Can you work these out from the model? Positions are in its coordinate system, mm. A direction names the side the tool comes from. Round coordinates to 2 decimals unless told otherwise and drop trailing zeros. Write each loop counter-clockwise with the first axis right and the second up, starting at its lowest first coordinate (ties: lowest second). Pieces come first, ordered by that corner, then holes. Notation, with made-up numbers: (2.5, 52.25) -> (39.5, 52.25) arc R11 cw to (39.5, 64.25) -> close; hole circle Ø10 at (50, 73). An arc over 180 degrees is marked (long way). Write item = value, one per line. Start each with the question number.
1) Imagine slicing it at B-B, the plane z = 0.9. State how many separate pieces and enclosed holes the cut face has, then the cut area to 3 significant figures.
2) If I drill on line 1 (Y direction, x = -1, z = 0.1); line 2 (Y direction, x = -15, z = 1.35); line 3 (Y direction, x = 9.25, z = 0.4), over which ranges is the centre line in solid material (lowest first)?
3) Imagine slicing it at A-A, the plane y = -13. Please give me the cut outline in (x, z) (3 decimals).
4) For faces 4 (the face through (8.4, -13.7, 1)), 5 (the face through (-0.2, -22.5, 1)), 6 (the face through (11.4, -12.7, 1)), which set-ups out of +Z, -Z, +X, -X, +Y, -Y let a thin tool reach every point of the face, with its end or its side?
5) I'm going to push flat-ended pins straight in: pin 1 (5 mm diameter, centred on x = -4, y = -16, fed in from +Z); pin 2 (3 mm diameter, centred on x = -15, y = -20, fed in from -Z). Where does each tip first touch, or does it pass through?
6) Thinking about a two-plate mould opening in X: for faces 1 (the face through (8.06, -0.91, 0.99)), 2 (the face through (-11.328, -12.604, 0.986)), 3 (the face through (0, -10, 0)), which applies, +X half, -X half, draft (parallel to the pull), parting line (faces both ways), or undercut?
from build123d import *

# Parameters (mm, degrees)
SKETCH_1_R         = 3
SKETCH_1_R_2       = 1
EXTRUDE_1_DEPTH    = 2
EXTRUDE_1_2_DEPTH  = 2
SKETCH_1_RX        = 12
SKETCH_1_RY        = 10.5
SKETCH_1_R_3       = 7.5
SKETCH_1_R_4       = 1.5
EXTRUDE_1_3_DEPTH  = 2
EXTRUDE_START      = -2
EXTRUDE_3_DEPTH    = 2
FILLET_3_R         = 1
EXTRUDE_4_DEPTH    = 2
HOLE_WIZARD_M3_1_D = 2.5


with BuildPart() as part:
    # Sketch 1 → Extrude 1 (new body)
    with BuildSketch(Plane.XY):
        with Locations((-15, -20)):
            Circle(SKETCH_1_R)
        with Locations((-15, -20)):
            Circle(SKETCH_1_R_2, mode=Mode.SUBTRACT)
    extrude(amount=EXTRUDE_1_DEPTH)



with BuildPart() as body_2:
    # Sketch 1 → Extrude 1 2 (new body)
    with BuildSketch(Plane.XY):
        with Locations(Location((15, -20, 0), (0, 0, 180))):
            Circle(SKETCH_1_R)
        with Locations(Location((15, -20, 0), (0, 0, 180))):
            Circle(SKETCH_1_R_2, mode=Mode.SUBTRACT)
    extrude(amount=EXTRUDE_1_2_DEPTH)


with BuildPart() as body_3:
    # Sketch 1 → Extrude 1 3 (new body)
    with BuildSketch(Plane.XY):
        with Locations((0, 0)):
            Ellipse(SKETCH_1_RX, SKETCH_1_RY)
        Circle(SKETCH_1_R_3, mode=Mode.SUBTRACT)
        with Locations((9.25, 0)):
            Circle(SKETCH_1_R_4, mode=Mode.SUBTRACT)
        with Locations(Location((-9.25, 0, 0), (0, 0, 180))):
            Circle(SKETCH_1_R_4, mode=Mode.SUBTRACT)
    extrude(amount=EXTRUDE_1_3_DEPTH)


with BuildPart() as part_1:
    add(part.part)

    add(body_2.part)  # Extrude 3 merges body 2

    add(body_3.part)  # Extrude 3 merges body 3
    # Sketch 7 → Extrude 3 (add)
    with BuildSketch(Plane.XY.offset(2).offset(EXTRUDE_START)):
        with BuildLine():
            Line((-7.838039348, -7.95071913), (-14.641154273, -17.021539031))
            ThreePointArc((-14.641154273, -17.021539031), (-13.2, -17.6), (-12.241154273, -18.821539031))
            Line((-12.241154273, -18.821539031), (-5.216878938, -9.455838584))
            add(Edge.make_bspline(
                [(-7.838039348, -7.95071913), (-6.640783086, -8.854377448), (-5.216878938, -9.455838584)],
                knots=[4.000625721, 4.000625721, 4.000625721, 4.262639533, 4.262639533, 4.262639533], degree=2, weights=[1, 0.991430862, 1]))
        make_face()
        with BuildLine():
            Line((5.216878938, -9.455838584), (12.241154273, -18.821539031))
            ThreePointArc((12.241154273, -18.821539031), (13.2, -17.6), (14.641154273, -17.021539031))
            Line((14.641154273, -17.021539031), (7.838039348, -7.95071913))
            add(Edge.make_bspline(
                [(5.216878938, -9.455838584), (6.640783086, -8.854377448), (7.838039348, -7.95071913)],
                knots=[2.020545775, 2.020545775, 2.020545775, 2.282559586, 2.282559586, 2.282559586], degree=2, weights=[1, 0.991430862, 1]))
        make_face()
        with BuildLine():
            ThreePointArc((-12.603200099, -21.804258915), (0, -22.5), (12.603200099, -21.804258915))
            ThreePointArc((12.603200099, -21.804258915), (12.022167048, -20.364020483), (12.239155559, -18.826229166))
            ThreePointArc((12.239155559, -18.826229166), (0, -19.5), (-12.239155559, -18.826229166))
            ThreePointArc((-12.239155559, -18.826229166), (-12.022167048, -20.364020483), (-12.603200099, -21.804258915))
        make_face()
    extrude(amount=EXTRUDE_3_DEPTH)

    # Fillet 3
    fillet_3_edges = [part_1.edges().sort_by_distance(p)[0] for p in [
        (-7.838039348, -7.95071913, 1),
        (7.838039348, -7.95071913, 1),
        (-14.641154273, -17.021539031, 1),
        (14.641154273, -17.021539031, 1),
        (12.603200099, -21.804258915, 1),
        (-12.603200099, -21.804258915, 1),
        (-5.216878938, -9.455838584, 1),
        (5.216878938, -9.455838584, 1),
    ]]
    fillet(fillet_3_edges, radius=FILLET_3_R)

    # Sketch 8 → Extrude 4 (add)
    with BuildSketch(Plane.XY.offset(2).offset(EXTRUDE_START)):
        with BuildLine():
            Line((-12.241154273, -18.821539031), (-11.183307296, -17.411076395))
            ThreePointArc((-11.183307296, -17.411076395), (-11.297779405, -18.415725331), (-10.477273878, -19.006651747))
            ThreePointArc((-10.477273878, -19.006651747), (-11.358572959, -18.919938786), (-12.239155559, -18.826229166))
            ThreePointArc((-12.239155559, -18.826229166), (-12.24015392, -18.823883674), (-12.241154273, -18.821539031))
        make_face()
        with BuildLine():
            Line((12.241154273, -18.821539031), (11.183307296, -17.411076395))
            ThreePointArc((11.183307296, -17.411076395), (11.297779405, -18.415725331), (10.477273878, -19.006651747))
            ThreePointArc((10.477273878, -19.006651747), (11.358572959, -18.919938786), (12.239155559, -18.826229166))
            ThreePointArc((12.239155559, -18.826229166), (12.24015392, -18.823883674), (12.241154273, -18.821539031))
        make_face()
    extrude(amount=EXTRUDE_4_DEPTH)

    # Hole Wizard M3 _1 (through all)
    with Locations(Plane(origin=(0, 0, 0), x_dir=(-1, 0, 0), z_dir=(0, 0, -1))):
        with Locations((-15, -20), (15, -20)):
            Hole(HOLE_WIZARD_M3_1_D / 2)


solid = part_1.part
Reported:
q1.separate_pieces = 1
q1.enclosed_holes = 6
q1.area = 394 mm²
q2.line_1 = -22.5 to -19.5, -10.46 to -7.43, 7.43 to 10.46
q2.line_2 = -23 to -21.25, -18.75 to -16.99
q2.line_3 = -22.13 to -19.12, -14.83 to -9.83, -6.69 to -1.5, 1.5 to 6.69
q3.outline = (-11.625, 0) -> (-7.875, 0) -> (-7.875, 2) -> (-11.625, 2) -> close; (7.875, 0) -> (11.625, 0) -> (11.625, 2) -> (7.875, 2) -> close
q4.face_4 = +Z, -Z
q4.face_5 = +Z, -Z, -Y
q4.face_6 = +Z, -Z, +X
q5.pin_1 = through
q5.pin_2 = 0
q6.face_1 = undercut
q6.face_2 = -X half
q6.face_3 = draft
